```python
from build123d import *

# Parameters (mm, degrees)
SKETCH_1_W             = 20
SKETCH_1_H             = 20
EXTRUDE_1_DEPTH        = 50
CUT_EXTRUDE_1_DEPTH    = 57.780278266
PATTERN_LINEAR_1_COUNT = 8
PATTERN_LINEAR_1_PITCH = 6.28


with BuildPart() as part:
    # 草图1 → 凸台-拉伸1 (new body)
    with BuildSketch(Plane.XY):
        with Locations((0, -8)):
            Rectangle(SKETCH_1_W, SKETCH_1_H)
    extrude(amount=EXTRUDE_1_DEPTH)

    # 草图2 → 切除-拉伸1 (cut, through all)
    with BuildSketch(Plane.ZY.offset(10)):
        with BuildLine():
            Line((0.842059531, 2), (2.360183044, -2.171010072))
            ThreePointArc((2.360183044, -2.171010072), (2.543241137, -2.409576022), (2.830029355, -2.5))
            Line((2.830029355, -2.5), (3.449970645, -2.5))
            ThreePointArc((3.449970645, -2.5), (3.736758863, -2.409576022), (3.919816956, -2.171010072))
            Line((3.919816956, -2.171010072), (5.437940469, 2))
            Line((5.437940469, 2), (0.842059531, 2))
        make_face()
    cut_extrude_1 = extrude(amount=-CUT_EXTRUDE_1_DEPTH, mode=Mode.SUBTRACT)

    # 阵列(线性)1: 切除-拉伸1 ×8
    with Locations(*[(0, 0, i * PATTERN_LINEAR_1_PITCH) for i in range(1, PATTERN_LINEAR_1_COUNT)]):
        add(cut_extrude_1, mode=Mode.SUBTRACT)


solid = part.part
```
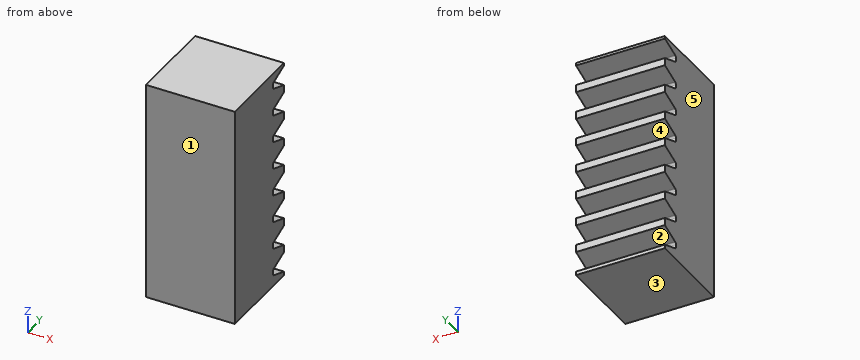
Here's how the part is built. I have some questions about the finished solid (model axes, mm). Face numbers are marked on the shaded views. A direction names the side the tool comes from. Coordinates: 2 decimals unless noted, no trailing zeros. Write each loop counter-clockwise with the first axis right and the second up, starting at its lowest first coordinate (ties: lowest second). Pieces come first, ordered by that corner, then holes. Notation, with made-up numbers: M -15,80 L 24,80 A20 cw 24,97 Z; hole C 51,6 d5. An arc over 180 degrees is marked long. Answer as CSV lines item,"result". Start each with the question number.
Q1. For the marked faces 1 and 2, which set-ups out of +Z, -Z, +X, -X, +Y, -Y let a thin tool reach every point of the face, with its end or its side?
Q2. Will these pins go through, and if not, where does the flat tip stop? pin 1 Ø0.7 at (x, z) = (1, 28) entering from +Y; pin 2 Ø0.7 at (x, z) = (-5, 34.5) entering from +Y; pin 3 Ø10 at (x, z) = (2.5, 42) entering from +Y.
Q3. Suppose I cut it at B-B, the plane z = 39.5. List the corners of the cut face in (x, y) for me.
Q4. I need wall thicknesses on probe 1 along Y at (x, z) = (9.25, 47.5); probe 2 along Y at (x, z) = (-1.75, 10). Which ranges of each line are inside material? Lowest first, please. Write a range as [from, to].
Q5. Suppose I cut it at A-A, the plane y = -1.25. State how many separate pieces and enclosed holes the cut face has, then the cut area to 3 significant figures.
Q6. If we mould it in two halves opening along Z, with no side actions, what happens to the marked faces 3, 4 and 5? For each: pulls with the +Z half, pulls with the -Z half, needs draft (parallel to the pull), parting line crosses it, or undercut.
Entries:
1,face 1,"+Z, -Z, +X, -X, -Y"
1,face 2,"+X, -X, +Y"
2,pin 1,"stops at y = -2.4"
2,pin 2,"stops at y = -2.49"
2,pin 3,"stops at y = 2"
3,outline,"M -10,-18 L 10,-18 L 10,-0.69 L -10,-0.69 Z"
4,probe 1,"y = [-18, -2.49]"
4,probe 2,"y = [-18, -2.42]"
5,separate pieces,"9"
5,enclosed holes,"0"
5,area,"643 mm²"
6,face 3,"pulls with the -Z half"
6,face 4,"undercut"
6,face 5,"needs draft"
